from build123d import *

# Parameters (mm, degrees)
F0_W     = 180
F0_H     = 180
F1_DEPTH = 10
F2_W     = 55
F2_H     = 55
F3_DEPTH = 40
F4_W     = 180
F4_H     = 180
F4_W_2   = 170
F4_H_2   = 170
F5_DEPTH = 83
F6_R     = 24.5
F7_DEPTH = 2
F8_R     = 42.5
F9_DEPTH = 5
F10_R    = 2.5
F11_R    = 2.5


with BuildPart() as f1:
    # F0 (on Top) → F1 (new body)
    with BuildSketch(Plane.XY):
        Rectangle(F0_W, F0_H)
    extrude(amount=F1_DEPTH)

    # F2 (on face) → F3 (join)
    with BuildSketch(Plane.XY.offset(10)):
        with Locations((0.5, 1.5)):
            Rectangle(F2_W, F2_H)
    extrude(amount=F3_DEPTH)

    # F4 (on face) → F5 (join)
    with BuildSketch(Plane.XY.offset(10)):
        Rectangle(F4_W, F4_H)
        Rectangle(F4_W_2, F4_H_2, mode=Mode.SUBTRACT)
    extrude(amount=F5_DEPTH)

    # F6 (on face) → F7 (cut)
    with BuildSketch(Plane.XY.offset(50)):
        with Locations((0.25, 2.5)):
            Circle(F6_R)
    extrude(amount=-F7_DEPTH, mode=Mode.SUBTRACT)

    # F8 (on face) → F9 (cut)
    with BuildSketch(Plane.XZ.offset(90)):
        with Locations((0, 46.5)):
            Circle(F8_R)
    extrude(amount=-F9_DEPTH, mode=Mode.SUBTRACT)

    # F10
    f10_edges = [f1.edges().sort_by_distance(p)[0] for p in [
        (90, 90, 46.5),
        (-90, 90, 46.5),
        (90, -90, 46.5),
        (-90, -90, 46.5),
    ]]
    fillet(f10_edges, radius=F10_R)

    # F11
    f11_edges = [f1.edges().sort_by_distance(p)[0] for p in [
        (-85, 85, 51.5),
        (85, 85, 51.5),
        (-85, -85, 51.5),
        (85, -85, 51.5),
    ]]
    fillet(f11_edges, radius=F11_R)


solid = f1.part
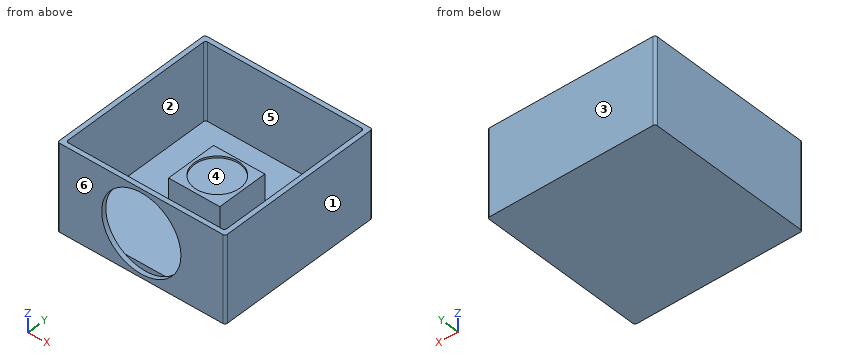
Check sheet for the modelled part. Datum: model origin and axes. Units: mm. Face numbers are marked on the shaded views. A direction names the side the tool comes from. Round coordinates to 2 decimals unless told otherwise and drop trailing zeros. Loops run counter-clockwise (first coordinate to the right, second up) from the corner with the lowest first, then second, coordinate; pieces in that order, holes last. Notation, with made-up numbers: M -18.75,10 L 29.25,10 A22 ccw 29.25,17 Z; hole C 43.5,2 d4. An arc over 180 degrees is marked long. One line per item, written item: value.
(1) Sectioned sample at D-D, the plane z = 82.5. Record the cut outline in (x, y).
Computed values:
outline: M -90,-87.5 A2.5 ccw -87.5,-90 L -22.59,-90 L -22.59,-85 L -82.5,-85 A2.5 cw -85,-82.5 L -85,82.5 A2.5 cw -82.5,85 L 82.5,85 A2.5 cw 85,82.5 L 85,-82.5 A2.5 cw 82.5,-85 L 22.59,-85 L 22.59,-90 L 87.5,-90 A2.5 ccw 90,-87.5 L 90,87.5 A2.5 ccw 87.5,90 L -87.5,90 A2.5 ccw -90,87.5 Z
(2) Sectioned sample at A-A, the plane y = 48. Record the cut outline in (x, z), then the cut area to 3 significant figures.
Computed values:
outline: M -90,0 L 90,0 L 90,93 L 85,93 L 85,10 L -85,10 L -85,93 L -90,93 Z
area: 2,630 mm^2
(3) Depth check by flat-ended pin: pin 1 Ø3 at (x, y) = (44, 43) entering from +Z; pin 2 Ø25 at (x, z) = (-1.5, 70) entering from -Y; pin 3 Ø14.5 at (x, y) = (-1.5, -2) entering from +Z. Enter the tip coordinate at first touch or a pass-through.
Computed values:
pin 1: stops at z = 10
pin 2: stops at y = 85
pin 3: stops at z = 48
(4) Thickness scan on line 1 (Y direction, x = 0.25, z = 48.75); line 2 (X direction, y = -5, z = 20.5); line 3 (Y direction, x = 22.5, z = 34). Record the ranges inside material, lowest first.
Computed values:
line 1: y = -26 to -22, 27 to 29, 85 to 90
line 2: x = -90 to -85, -27 to 28, 85 to 90
line 3: y = -26 to 29, 85 to 90
(5) Access from +Z, -Z, +X, -X, +Y, -Y to the whole of each face (thin tool, end or side, straight path). Record for the marked faces 5 and 6.
Computed values:
face 5: +Z
face 6: +Z, -Z, +X, -X, -Y
(6) Release check for a two-part mould opening along Y. For the marked faces 1, 2, 3 and 4 record: +Y half, -Y half, draft (parallel to the pull), parting line (faces both ways), or undercut.
Computed values:
face 1: draft
face 2: undercut
face 3: +Y half
face 4: undercut
(7) Sectioned sample at B-B, the plane x = -34.5. Record the cut outline in (y, z), then the cut area to 3 significant figures.
Computed values:
outline: M -90,0 L 90,0 L 90,93 L 85,93 L 85,10 L -85,10 L -85,21.68 L -90,21.68 Z; M -90,71.32 L -85,71.32 L -85,93 L -90,93 Z
area: 2,380 mm^2
